Design review of the part built by this model. Coordinates are the model's own, in mm. A direction names the side the tool comes from. Coordinates: 2 decimals unless noted, no trailing zeros. Order: outer loops, then holes, each group sorted by start corner. A loop starts at its lowest first (then second) coordinate and runs counter-clockwise, first axis right, second up. Notation, with made-up numbers: (12, 31) -> (69, 31) arc R21 ccw to (69, 43) -> close; hole circle Ø6 at (53, -25). An arc over 180 degrees is marked (long way). Use a Markdown table: item, result. Add a question column.
Q1. Add section A-A (x = 157). State the section outline as (y, z) points.
Q2. Add section C-C (z = 16). State the section outline as (x, y) points.
Q3. The part is to be moulded in two halves that separate along X. For faces 5 (the face through (156, 5.95, -4)), 6 (the face through (36.63, 2.46, -4.7)), 7 (the face through (103, 3.5, -2)), say which applies: pulls with the +X half, pulls with the -X half, needs draft (parallel to the pull), parting line crosses it, or undercut.
Q4. Machinability: for faces 1 (the face through (67, 3.5, 5)), 2 (the face through (108, 2, 0)), 3 (the face through (1.82, 0.99, 4.1)), 4 (the face through (59, 5, -5)), which of the approach directions +Z, -Z, +X, -X, +Y, -Y give a long, thin tool a straight path to every point of the face, cutting with its end or side? Answer none if there is none.
Q5. Insertion check: pin 1 (0.8 mm diameter, centred on y = 5.5, z = -6.5, fed in from -X); pin 2 (5 mm diameter, centred on x = 76.5, z = -6.5, fed in from +Y); pin 3 (1 mm diameter, centred on y = 1, z = 8.5, fed in from +X); pin 4 (1.5 mm diameter, centred on x = 38, z = 9.5, fed in from -Y). Each pin has a flat end and moves straight along its axis. Give the tip position at first contact, or say it passes through.
Q6. Add section B-B (x = 64.5). State the section outline as (y, z) points.
Q7. Wall thickness on probe 1 along Z at (x, y) = (71, 2); probe 2 along Z at (x, y) = (54, 2.8); probe 3 along X at (y, z) = (3.85, -1): over which ranges is each line inside the solid? List them lowest first.
from build123d import *

# Parameters (mm, degrees)
SKETCH_1_R          = 1.525
EXTRUDE_2_DEPTH     = 5
CUT_EXTRUDE_START   = 3.5
CUT_EXTRUDE_1_DEPTH = 158.761433703
EXTRUDE_START       = -5
EXTRUDE_4_DEPTH     = 5.95
SKETCH_4_R          = 1.525
CUT_EXTRUDE_2_DEPTH = 162.293684005
SKETCH_5_R          = 3
CUT_EXTRUDE_3_DEPTH = 2
FILLET_1_R          = 4.5
CUT_EXTRUDE_4_DEPTH = 162.293684005
FILLET_4_R          = 0.5
FILLET_5_R          = 2
FILLET_11_R         = 1
CUT_EXTRUDE_5_DEPTH = 10
FILLET_12_R         = 2


with BuildPart() as part:
    # 草图1 → 凸台-拉伸2 (new body)
    with BuildSketch(Plane(origin=(0, 0, 0), x_dir=(1, 0, 0), z_dir=(0, 1, 0))):
        with BuildLine():
            Line((0, 0), (33.333333333, 0))
            Line((33.333333333, 0), (40, 9.5))
            Line((40, 9.5), (44, 9.5))
            Line((44, 9.5), (54, 9.5))
            Line((54, 9.5), (154, 9.5))
            Line((154, 9.5), (160, 4.5))
            Line((160, 4.5), (160, 0))
            Line((160, 0), (54.433012702, 0))
            ThreePointArc((54.433012702, 0), (53.5, -0.25), (54.433012702, -0.5))
            Line((54.433012702, -0.5), (67, -0.5))
            Line((67, -0.5), (70, -0.5))
            Line((70, -0.5), (79.5, -0.5))
            Line((79.5, -0.5), (79.5, -9.5))
            Line((79.5, -9.5), (70, -9.5))
            Line((70, -9.5), (69, -9.5))
            Line((69, -9.5), (69, -10.3))
            Line((69, -10.3), (61, -10.3))
            Line((61, -10.3), (61, -9.5))
            Line((61, -9.5), (20.55, -9.5))
            Line((20.55, -9.5), (20.55, -19.5))
            Line((20.55, -19.5), (14, -19.5))
            Line((14, -19.5), (14, -9.5))
            Line((14, -9.5), (0, -9.5))
            Line((0, -9.5), (0, 0))
        make_face()
        with Locations(Location((4.75, -4.75, 0), (0, 0, 270))):
            Circle(SKETCH_1_R, mode=Mode.SUBTRACT)
    extrude(amount=EXTRUDE_2_DEPTH)

    # 草图2 → 切除-拉伸1 (cut, through all)
    with BuildSketch(Plane(origin=(0, 0, 0), x_dir=(1, 0, 0), z_dir=(0, 1, 0)).offset(CUT_EXTRUDE_START)):
        Polygon((54, -9.5), (54, -0.5), (67, -0.5), (83.595743226, -0.5), (83.595743226, -15.95528926), (54, -15.95528926), align=None)
        Polygon((54, 0), (154, 0), (152, 4.5), (56, 4.5), align=None)
    extrude(amount=CUT_EXTRUDE_1_DEPTH, mode=Mode.SUBTRACT)

    # 草图3 → 凸台-拉伸4 (add)
    with BuildSketch(Plane(origin=(0, 5, 0), x_dir=(1, 0, 0), z_dir=(0, 1, 0)).offset(EXTRUDE_START)):
        Polygon((152, 4.5), (152, 9.5), (154, 9.5), (160, 4.5), (160, 0), (154, 0), align=None)
    extrude(amount=EXTRUDE_4_DEPTH)

    # 草图4 → 切除-拉伸2 (cut, through all)
    with BuildSketch(Plane.XY):
        with Locations((157, 2.975)):
            Circle(SKETCH_4_R)
    extrude(amount=-CUT_EXTRUDE_2_DEPTH, mode=Mode.SUBTRACT)

    # 草图5 → 切除-拉伸3 (cut)
    with BuildSketch(Plane(origin=(0, 0, 0), x_dir=(1, 0, 0), z_dir=(0, 1, 0))):
        with Locations(Location((4.75, -4.75, 0), (0, 0, 270))):
            Circle(SKETCH_5_R)
    extrude(amount=CUT_EXTRUDE_3_DEPTH, mode=Mode.SUBTRACT)

    # 圆角1
    fillet_1_edges = [part.edges().sort_by_distance(p)[0] for p in [
        (0, 2.5, 9.5),
        (0, 2.5, 0),
    ]]
    fillet(fillet_1_edges, radius=FILLET_1_R)

    # 草图7 → 切除-拉伸4 (cut, through all)
    with BuildSketch(Plane(origin=(0, 0, 0), x_dir=(0, 0, -1), z_dir=(1, 0, 0))):
        Polygon((-19.5, 2.5), (-12, 5), (-19.5, 5), align=None)
    extrude(amount=CUT_EXTRUDE_4_DEPTH, mode=Mode.SUBTRACT)

    # 圆角4
    fillet_4_edges = [part.edges().sort_by_distance(p)[0] for p in [
        (20.55, 1.25, 19.5),
        (14, 1.25, 19.5),
        (17.275, 2.5, 19.5),
    ]]
    fillet(fillet_4_edges, radius=FILLET_4_R)

    # 圆角5
    fillet_5_edges = [part.edges().sort_by_distance(p)[0] for p in [
        (33.333333333, 2.5, 0),
        (40, 2.5, -9.5),
    ]]
    fillet(fillet_5_edges, radius=FILLET_5_R)

    # 圆角11
    # the kernel refuses this fillet: 1 mm, written as the material it adds along each edge
    with BuildSketch(Plane(origin=(61, 0, 9.5), x_dir=(-1, 0, 0), z_dir=(0, 1, 0))) as fillet_11_piece_1:
        with BuildLine():
            CenterArc((0.979795897, 1), FILLET_11_R, 191.536959033, 78.463040967)
            Line((0, 0.8), (-0.019595918, 0.796))
            ThreePointArc((-0.019595918, 0.796), (-0.02, 0.4), (-0.02, 0))
            Line((-0.02, 0), (0, -0.02))
            Line((0, -0.02), (0.979795897, -0.02))
            Line((0.979795897, -0.02), (0.979795897, 0))
        make_face()
    extrude(amount=3.5)

    # 草图9 → 切除-拉伸5 (cut)
    with BuildSketch(Plane(origin=(0, 0, 0), x_dir=(1, 0, 0), z_dir=(0, 1, 0))):
        Polygon((75, -0.5), (79.5, -5), (79.5, -0.5), align=None)
    extrude(amount=CUT_EXTRUDE_5_DEPTH, mode=Mode.SUBTRACT)

    # 圆角12
    fillet_12_edges = [part.edges().sort_by_distance(p)[0] for p in [
        (75, 1.75, 0.5),
        (79.5, 1.75, 5),
    ]]
    fillet(fillet_12_edges, radius=FILLET_12_R)


solid = part.part
Established:
| question | item | result |
|---|---|---|
| 1 | outline | (0, -7) -> (1.45, -7) -> (1.45, 0) -> (0, 0) -> close; (4.5, -7) -> (5.95, -7) -> (5.95, 0) -> (4.5, 0) -> close |
| 2 | outline | (14, 0) -> (20.55, 0) -> (20.55, 3.67) -> (14, 3.67) -> close |
| 3 | face 5 | needs draft |
| 3 | face 6 | pulls with the -X half |
| 3 | face 7 | undercut |
| 4 | face 1 | +Z, +X, +Y |
| 4 | face 2 | +X, +Y, -Y |
| 4 | face 3 | -Y |
| 4 | face 4 | +Z, -Z, -X, +Y |
| 5 | pin 1 | x = 152 |
| 5 | pin 2 | y = 5 |
| 5 | pin 3 | x = 79.5 |
| 5 | pin 4 | y = 0 |
| 6 | outline | (0, -9.5) -> (5, -9.5) -> (5, -4.5) -> (3.5, -4.5) -> (3.5, 0) -> (0, 0) -> close; (0, 0.5) -> (3.5, 0.5) -> (3.5, 10.3) -> (0, 10.3) -> close |
| 7 | probe 1 | -9.5 to 0, 0.5 to 9.5 |
| 7 | probe 2 | -9.5 to -0.25, 0.75 to 9.5 |
| 7 | probe 3 | 34.04 to 54.44, 153.56 to 155.75, 158.25 to 160 |
